Verification items for this drawing (mm, ordinates from the low corner). A direction names the side the tool comes from. Round coordinates to 2 decimals unless told otherwise and drop trailing zeros. Loops run counter-clockwise (first coordinate to the right, second up) from the corner with the lowest first, then second, coordinate; pieces in that order, holes last. Notation, with made-up numbers: M 14,84.5 L 33,84.5 A17 ccw 33,96.5 Z; hole C -29.5,-29 d7. An arc over 180 degrees is marked long. Answer as CSV lines item,"result".
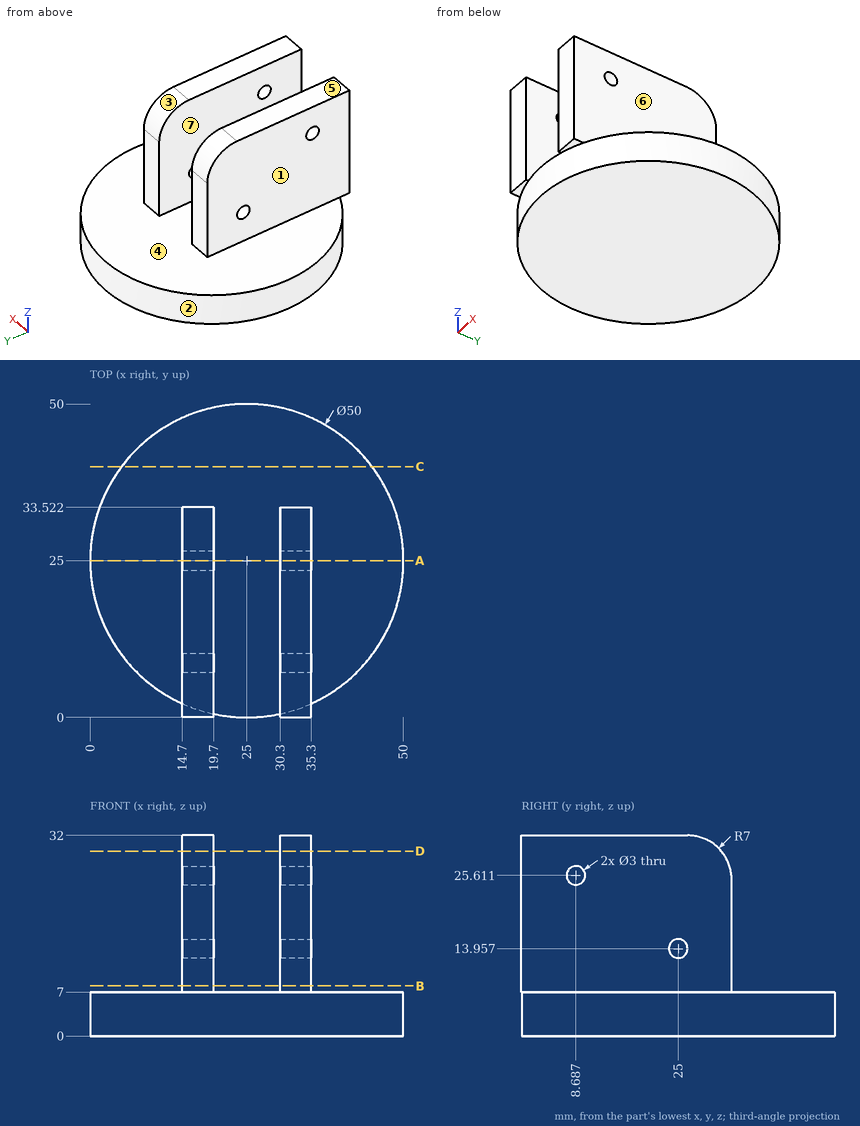
1) Section check D-D (z = 29.5). Record the cut outline in (x, y).
Here are the results:
outline,"M 14.7,0 L 19.7,0 L 19.7,31.88 L 14.7,31.88 Z; M 30.3,0 L 35.3,0 L 35.3,31.88 L 30.3,31.88 Z"
2) Section check A-A (y = 25). Record the cut outline in (x, z), plus the area to 3 significant figures.
Here are the results:
outline,"M 0,0 L 50,0 L 50,7 L 35.3,7 L 35.3,12.46 L 30.3,12.46 L 30.3,7 L 19.7,7 L 19.7,12.46 L 14.7,12.46 L 14.7,7 L 0,7 Z; M 14.7,15.46 L 19.7,15.46 L 19.7,32 L 14.7,32 Z; M 30.3,15.46 L 35.3,15.46 L 35.3,32 L 30.3,32 Z"
area,"570 mm^2"
3) Set-up check for the marked faces 5, 6 and 7: record each of +Z, -Z, +X, -X, +Y, -Y from which the full face is reachable in a straight line by a thin tool's end or side.
Here are the results:
face 5,"+Z, +X, -X, +Y, -Y"
face 6,"+Z, +X, +Y, -Y"
face 7,"+Z, +Y, -Y"
4) Draft check along X on the marked faces 1, 2, 3 and 4. Enter one of: +X half, -X half, draft (parallel to the pull), parting line (faces both ways), or undercut.
Here are the results:
face 1,"-X half"
face 2,"parting line"
face 3,"draft"
face 4,"undercut"
5) Go/stop test with flat-tipped pins: pin 1 (6 mm diameter, centred on y = 29.5, z = 17.5, fed in from +X); pin 2 (1 mm diameter, centred on x = 21.5, y = 35, fed in from +Z); pin 3 (5 mm diameter, centred on y = 8.69, z = 25.61, fed in from -X); pin 4 (2.5 mm diameter, centred on y = 25, z = 13.96, fed in from +X). Record where each tip stops, or that it passes through.
Here are the results:
pin 1,"stops at x = 35.3"
pin 2,"stops at z = 7"
pin 3,"stops at x = 14.7"
pin 4,"passes through"
6) Material ranges on probe 1 along X at (y, z) = (21, 28); probe 2 along Z at (x, y) = (5, 24); probe 3 along Y at (x, z) = (34, 16), recorded low to high.
Here are the results:
probe 1,"x = 14.7 to 19.7, 30.3 to 35.3"
probe 2,"z = 0 to 7"
probe 3,"y = 0 to 33.52"
7) Section check C-C (y = 40). Record the cut outline in (x, z).
Here are the results:
outline,"M 5,0 L 45,0 L 45,7 L 5,7 Z"
8) Section check B-B (z = 8). Record the cut outline in (x, y), plus the area to 3 significant figures.
Here are the results:
outline,"M 14.7,0 L 19.7,0 L 19.7,33.52 L 14.7,33.52 Z; M 30.3,0 L 35.3,0 L 35.3,33.52 L 30.3,33.52 Z"
area,"335 mm^2"
